The figure shows three views and two pictorial views of one solid part (mm, origin at its lowest corner). Answer the questions. A direction names the side the tool comes from. Coordinates: 2 decimals unless noted, no trailing zeros. Loops run counter-clockwise (first coordinate to the right, second up) from the corner with the lowest first, then second, coordinate; pieces in that order, holes last. Notation, with made-up numbers: (5.5, -32) -> (21.5, -32) arc R12 cw to (21.5, -23) -> close; hole circle Ø1 at (6, -33.75). An arc over 180 degrees is marked (long way). Use a Markdown table: item, result. Add a question column.
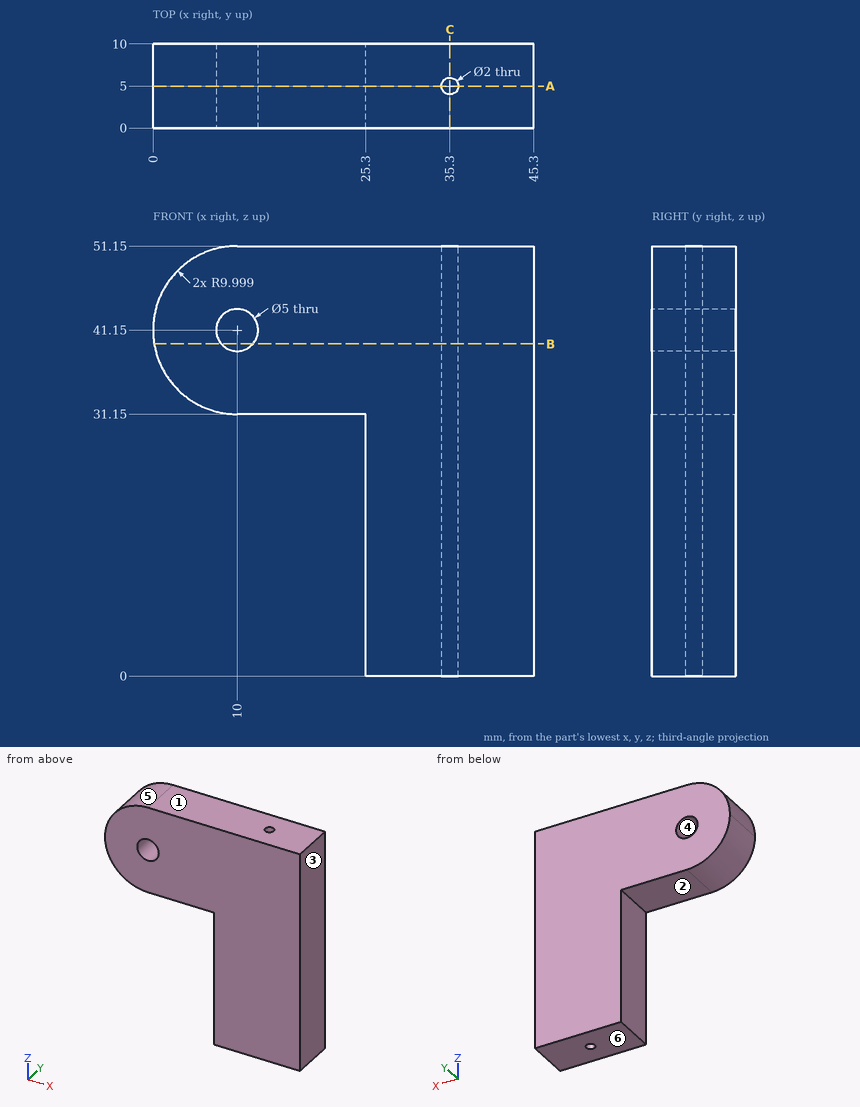
Item 1: Section A-A (y = 5) is taken. Count the separate pieces of the cut face and the enclosed holes in it, then the cut area to 3 significant figures.
Item 2: Find the intervals of material crossed by probe 1 along Z at (x, y) = (10, 4.5); probe 2 along Y at (x, z) = (35.3, 34); probe 3 along X at (y, z) = (5, 11), in increasing order.
Item 3: For a pull along Z with two mould halves and no side action, classify the marked faces 3, 4, 5 and 6 as +Z half, -Z half, draft (parallel to the pull), parting line (faces both ways), or undercut.
Item 4: Section B-B (z = 39.5) is taken. Determine the outline of the cut face in (x, y), then the cut area to 3 significant figures.
Item 5: Section C-C (x = 35.3) is taken. Determine the outline of the cut face in (y, z), then the cut area to 3 significant figures.
Item 6: For the marked faces 1 and 2, determine the directions among +Z, -Z, +X, -X, +Y, -Y from which every point of the face is accessible in a straight line to the end or side of a thin tool.
Item 7: Given pin 1 (1.8 mm diameter, centred on x = 35.3, y = 5, fed in from +Z) (3 decimals), flat-ended and moving along its own axis, determine where the tip first touches the part or whether it passes through.
Output:
| question | item | result |
|---|---|---|
| 1 | separate pieces | 2 |
| 1 | enclosed holes | 1 |
| 1 | area | 1,360 mm2 |
| 2 | probe 1 | z = 31.15 to 38.65, 43.65 to 51.15 |
| 2 | probe 2 | y = 0 to 4, 6 to 10 |
| 2 | probe 3 | x = 25.3 to 34.3, 36.3 to 45.3 |
| 3 | face 3 | draft |
| 3 | face 4 | undercut |
| 3 | face 5 | +Z half |
| 3 | face 6 | -Z half |
| 4 | outline | (0.14, 0) -> (8.12, 0) -> (8.12, 10) -> (0.14, 10) -> close; (11.88, 0) -> (45.3, 0) -> (45.3, 10) -> (11.88, 10) -> close; hole circle Ø2 at (35.3, 5) |
| 4 | area | 411 mm2 |
| 5 | outline | (0, 0) -> (4, 0) -> (4, 51.15) -> (0, 51.15) -> close; (6, 0) -> (10, 0) -> (10, 51.15) -> (6, 51.15) -> close |
| 5 | area | 409 mm2 |
| 6 | face 1 | +Z, +X, -X, +Y, -Y |
| 6 | face 2 | -Z, -X, +Y, -Y |
| 7 | pin 1 | passes through |
